from build123d import *

# Parameters (mm, degrees)
SKETCH_R      = 8
PAD_DEPTH     = 5
PAD001_DEPTH  = 20
SKETCH002_R   = 10
SKETCH002_R_2 = 6
PAD002_DEPTH  = 2


with BuildPart() as part:
    # Sketch → Pad (new body)
    with BuildSketch(Plane.XY):
        with BuildLine():
            ThreePointArc((-2.142857, -9.76771), (10, 0), (-2.142857, 9.76771))
            Line((-28.857143, 3.907084), (-2.142857, 9.76771))
            ThreePointArc((-28.857143, 3.907084), (-32, 0), (-28.857143, -3.907084))
            Line((-2.142857, -9.76771), (-28.857143, -3.907084))
        make_face()
        Circle(SKETCH_R, mode=Mode.SUBTRACT)
    extrude(amount=PAD_DEPTH)

    # Sketch001 (on Face7 of Pad) → Pad001 (join)
    with BuildSketch(Plane.XY.offset(5)):
        with BuildLine():
            ThreePointArc((-28.857143, 3.907084), (-32, -1.3e-05), (-28.857117, -3.90709))
            Line((-24, -4.972619), (-28.857117, -3.90709))
            Line((-24, -4.972619), (-24, 4.972653))
            Line((-24, 4.972653), (-28.857143, 3.907084))
        make_face()
    extrude(amount=PAD001_DEPTH)

    # Sketch002 → Pad002 (join)
    with BuildSketch(Plane(origin=(0, 0, 0), x_dir=(1, 0, 0), z_dir=(0, 0, -1))):
        Circle(SKETCH002_R)
        Circle(SKETCH002_R_2, mode=Mode.SUBTRACT)
    extrude(amount=PAD002_DEPTH)


solid = part.part
Here's how the part is built. I have some questions about the finished solid (model axes, mm). A direction names the side the tool comes from. Round coordinates to 2 decimals unless told otherwise and drop trailing zeros. Write each loop counter-clockwise with the first axis right and the second up, starting at its lowest first coordinate (ties: lowest second). Pieces come first, ordered by that corner, then holes.
1. Suppose I cut it at D-D (y = 7.25). List the corners of the cut face in (x, z) for me, and give its area (3 significant figures).
2. Suppose I cut it at A-A (y = 0). List the corners of the cut face in (x, z) for me, and give its area (3 significant figures).
3. For faces 1 (the flat face through (-15.687, 6.796, 2.465)), 2 (the flat face through (-10, 0, 5)), which set-ups out of +Z, -Z, +X, -X, +Y, -Y let a thin tool reach every point of the face, with its end or its side?
4. Will these pins go through, and if not, where does the flat tip stop? pin 1 Ø10 at (x, y) = (4.5, -3.5) entering from +Z; pin 2 Ø3 at (x, z) = (-23, 16.5) entering from -Y; pin 3 Ø0.9 at (x, y) = (-27, 4.5) entering from -Z.
5. If we mould it in two halves opening along X, with no side actions, what happens to faces 3 (the cylindrical face through (-1.73, -7.81, 2.46)), 4 (the flat face through (-27, 0, 25)), 5 (the flat face through (-26.39, 4.45, 14.86)), 6 (the flat face through (-2, -6, 0))? For each: released by +X, released by -X, zero draft, split by the parting line, or undercut.
6. I need wall thicknesses on L1, parallel to Y at x = 0, z = 1.6; L2, parallel to X at y = 0, z = -1.2; L3, parallel to Z at x = 7.5, y = 1. Which ranges of each line are inside material? Lowest first, please.
7. Suppose I cut it at B-B (x = 0). List the corners of the cut face in (y, z) for me.
8. Suppose I cut it at C-C (z = 3.75). List the corners of the cut face in (x, y) for me.
Answer sheet:
1. outline: (-13.62, 0) - (-6.89, 0) - (-6.89, -2) - (6.89, -2) - (6.89, 5) - (3.38, 5) - (3.38, 0) - (-3.38, 0) - (-3.38, 5) - (-13.62, 5) - close
1. area: 96.3 mm2
2. outline: (-32, 0) - (-10, 0) - (-10, -2) - (-6, -2) - (-6, 0) - (-8, 0) - (-8, 5) - (-24, 5) - (-24, 25) - (-32, 25) - close; (6, -2) - (10, -2) - (10, 5) - (8, 5) - (8, 0) - (6, 0) - close
2. area: 306 mm2
3. face 1: +Z, -Z, -X, +Y
3. face 2: +Z, +X, +Y, -Y
4. pin 1: stops at z = 5
4. pin 2: stops at y = -4.97
4. pin 3: stops at z = 0
5. face 3: undercut
5. face 4: zero draft
5. face 5: released by -X
5. face 6: undercut
6. L1: y = -10 to -8, 8 to 10
6. L2: x = -10 to -6, 6 to 10
6. L3: z = -2 to 0
7. outline: (-10, -2) - (-6, -2) - (-6, 0) - (-8, 0) - (-8, 5) - (-10, 5) - close; (6, -2) - (10, -2) - (10, 5) - (8, 5) - (8, 0) - (6, 0) - close
8. outline: (-28.86, -3.91) - (-2.14, -9.77) arc R10 ccw (long way) to (-2.14, 9.77) - (-28.86, 3.91) arc R4 ccw to start; hole circle Ø16 at (0, 0)
